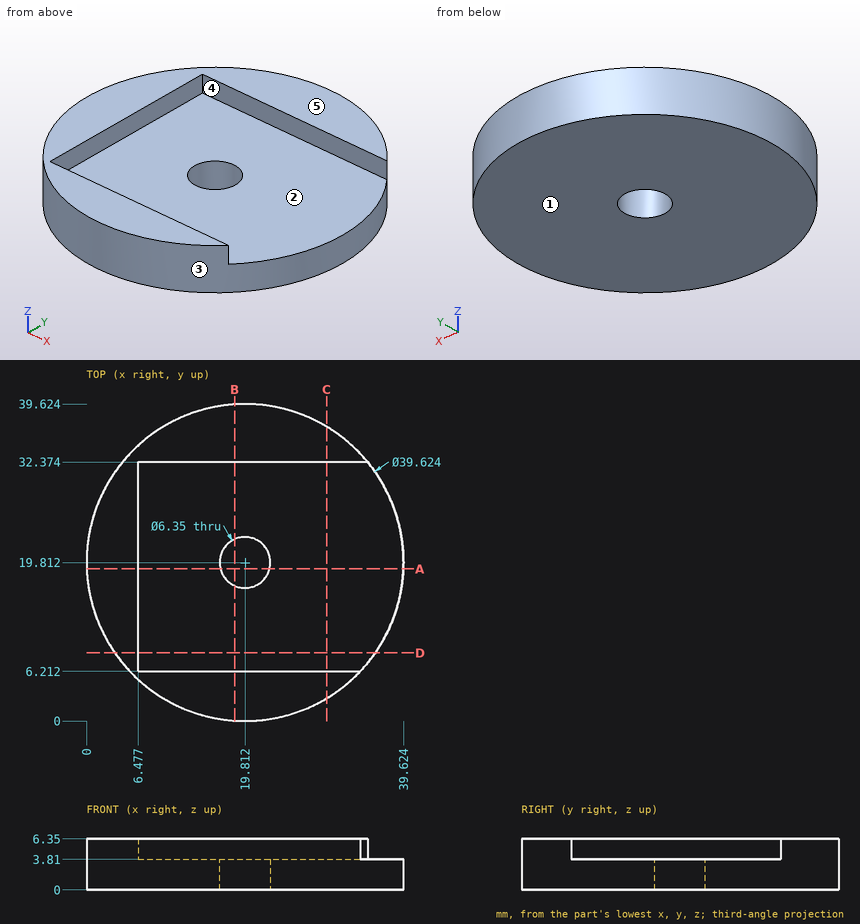
Source: three-view drawing plus pictorial views. Frame: mm from the lowest corner of the part. A direction names the side the tool comes from. Give positions to 0.01 mm unless a question says otherwise; leave off trailing zeros. Write each loop counter-clockwise with the first axis right and the second up, starting at its lowest first coordinate (ties: lowest second). Pieces come first, ordered by that corner, then holes. Notation, with made-up numbers: (18, -15.75) - (41, -15.75) arc R12 cw to (41, 4.25) - close; hole circle Ø9 at (11, -27.5). An arc over 180 degrees is marked (long way). Write item = value, one per line. Start each with the question number.
Q1. Pin query (flat end, axial travel): pin 1 Ø3 at (x, z) = (18, 4) entering from -Y; pin 2 Ø1.5 at (y, z) = (30.5, 1) entering from +X; pin 3 Ø3 at (y, z) = (14.5, 4.5) entering from +X. Return the tip coordinate at first contact, or that it passes through.
Q2. Draft query along Y for the marked faces 1, 2 and 3. Return one class per face: +Y half, -Y half, draft (parallel to the pull), parting line (faces both ways), or undercut.
Q3. Reachability of the marked faces 4 and 5 from +Z, -Z, +X, -X, +Y, -Y: full face, straight path, thin tool, end or side. Return the list, or none.
Q4. Material intervals for probe 1 along Z at (x, y) = (15.5, 19.5); probe 2 along X at (y, z) = (18, 3.5) (1 decimal); probe 3 along Y at (x, z) = (25.5, 4.25) (1 decimal), sorted ascending.
Q5. Cut plane B-B, the plane x = 18.5. Return loops of the section in (y, z), then the cut area to 3 significant figures.
Q6. Cut plane A-A, the plane y = 19. Return loops of the section in (x, z).
Q7. Cut plane D-D, the plane y = 8.5. Return loops of the section in (x, z), then the cut area to 3 significant figures.
Q8. Cut plane C-C, the plane x = 30. Return loops of the section in (y, z).
Computed values:
q1.pin_1 = 0
q1.pin_2 = 36.95
q1.pin_3 = 39.22
q2.face_1 = draft
q2.face_2 = undercut
q2.face_3 = parting line
q3.face_4 = +Z, +X
q3.face_5 = +Z, +X, -X, +Y, -Y
q4.probe_1 = 0 to 3.81
q4.probe_2 = 0.1 to 17.2, 22.4 to 39.5
q4.probe_3 = 0.8 to 6.2, 32.4 to 38.8
q5.outline = (0.04, 0) - (16.92, 0) - (16.92, 3.81) - (6.21, 3.81) - (6.21, 6.35) - (0.04, 6.35) - close; (22.7, 0) - (39.58, 0) - (39.58, 6.35) - (32.37, 6.35) - (32.37, 3.81) - (22.7, 3.81) - close
q5.area = 163 mm²
q6.outline = (0.02, 0) - (16.74, 0) - (16.74, 3.81) - (6.48, 3.81) - (6.48, 6.35) - (0.02, 6.35) - close; (22.88, 0) - (39.61, 0) - (39.61, 3.81) - (22.88, 3.81) - close
q7.outline = (3.55, 0) - (36.08, 0) - (36.08, 3.81) - (6.48, 3.81) - (6.48, 6.35) - (3.55, 6.35) - close
q7.area = 131 mm²
q8.outline = (2.82, 0) - (36.8, 0) - (36.8, 6.35) - (32.37, 6.35) - (32.37, 3.81) - (6.21, 3.81) - (6.21, 6.35) - (2.82, 6.35) - close
